For this review, take the finished solid that the model builds, in its own axes (mm). A direction names the side the tool comes from. Round coordinates to 2 decimals unless told otherwise and drop trailing zeros. Write each loop counter-clockwise with the first axis right and the second up, starting at its lowest first coordinate (ties: lowest second). Pieces come first, ordered by that corner, then holes.
from build123d import *

# Parameters (mm, degrees)
F1_DEPTH = 50.8
F2_DEPTH = 18.288
F3_DEPTH = 6.35
F0_W     = 25.4
F0_H     = 38.6286331601
F5_R     = 5.08


with BuildPart() as f1:
    # F0 (on Front) → F1 (new body, symmetric)
    with BuildSketch(Plane.XZ):
        Polygon((38.1, -12.7), (38.1, 12.7), (16.5100004677, 12.7), (-30.6439399719, 12.7), (-38.1, 12.7), (-38.1, -12.7), align=None)
    extrude(amount=F1_DEPTH, both=True)

    # F0 (on Front) → F2 (join, symmetric)
    with BuildSketch(Plane.XZ):
        with BuildLine():
            Line((16.5100004677, 12.7), (38.1, 12.7))
            Line((38.1, 12.7), (38.1, 24.0545344999))
            ThreePointArc((38.1, 24.0545344999), (39.9923105597, 28.6229763174), (44.5607523772, 30.5152868771))
            Line((44.5607523772, 30.5152868771), (51.4560379088, 30.5152868771))
            Line((51.4560379088, 30.5152868771), (51.4560379088, 52.1052864094))
            Line((51.4560379088, 52.1052864094), (44.5607523772, 52.1052864094))
            ThreePointArc((44.5607523772, 52.1052864094), (24.7258754846, 43.8894113925), (16.5100004677, 24.0545344999))
            Line((16.5100004677, 24.0545344999), (16.5100004677, 12.7))
        make_face()
        Polygon((51.4560379088, 52.1052864094), (51.4560379088, 30.5152868771), (64.020066675, 30.5152868771), (64.020066675, 52.1052864094), (58.4391281009, 52.1052864094), align=None)
    extrude(amount=F2_DEPTH, both=True)

    # F0 (on Front) → F3 (join, symmetric)
    with BuildSketch(Plane.XZ):
        with BuildLine():
            Line((-30.6439399719, 12.7), (16.5100004677, 12.7))
            Line((16.5100004677, 12.7), (16.5100004677, 24.0545344999))
            ThreePointArc((16.5100004677, 24.0545344999), (24.7258754846, 43.8894113925), (44.5607523772, 52.1052864094))
            Line((44.5607523772, 52.1052864094), (51.4560379088, 52.1052864094))
            Line((51.4560379088, 52.1052864094), (51.4560379088, 56.1626598461))
            add(Edge.make_bspline(
                [(51.4560379088, 56.1626598461), (40.4668177648, 57.3816540823), (15.1828966136, 61.2777253632), (-18.425734597, 32.7653036797), (-26.9961953148, 18.7397968243), (-30.6439399719, 12.7)],
                knots=[0.062706619, 0.062706619, 0.062706619, 0.062706619, 0.3573556866, 0.7280176576, 1, 1, 1, 1], degree=3))
        make_face()
        with BuildLine():
            add(Edge.make_bspline(
                [(58.4391281009, 55.5037148297), (56.1240075207, 55.6667510787), (53.7947415268, 55.9032359568), (51.4560379088, 56.1626598461)],
                knots=[0, 0, 0, 0, 0.062706619, 0.062706619, 0.062706619, 0.062706619], degree=3))
            Line((51.4560379088, 56.1626598461), (51.4560379088, 52.1052864094))
            Line((51.4560379088, 52.1052864094), (58.4391281009, 52.1052864094))
            Line((58.4391281009, 52.1052864094), (58.4391281009, 55.5037148297))
        make_face()
    extrude(amount=F3_DEPTH, both=True)

    # F0 (on Front) → F4 (revolve)
    with BuildSketch(Plane.XZ):
        with Locations((89.5560379088, 39.5638855255)):
            Rectangle(F0_W, F0_H)
    revolve(axis=Axis((76.8560379088, 0, 39.5638855255), (0, 0, -1)))

    # F5
    f5_edges = [f1.edges().sort_by_distance(p)[0] for p in [
        (-38.1, 0, 12.7),
        (0, -50.8, 12.7),
        (38.1, -34.544, 12.7),
        (38.1, -50.8, 0),
        (-38.1, -50.8, 0),
        (38.1, 34.544, 12.7),
        (38.1, 50.8, 0),
        (0, 50.8, 12.7),
        (-38.1, 50.8, 0),
    ]]
    fillet(f5_edges, radius=F5_R)


solid = f1.part
(1) We need section A-A, the plane z = 0. Give the boundary of the cut face in (x, y).
Geometry check:
outline: (-38.1, -45.72) arc R5.08 ccw to (-33.02, -50.8) - (33.02, -50.8) arc R5.08 ccw to (38.1, -45.72) - (38.1, 45.72) arc R5.08 ccw to (33.02, 50.8) - (-33.02, 50.8) arc R5.08 ccw to (-38.1, 45.72) - close
(2) For pin 1 Ø4 at (x, z) = (73.5, 42) entering from -Y; pin 2 Ø22.5 at (x, z) = (23, 38.5) entering from +Y; pin 3 Ø2 at (y, z) = (2.5, -2) entering from +X, all flat-tipped, find the tip position at first contact; note any pin that passes through.
Geometry check:
pin 1: stops at y = -25.36
pin 2: stops at y = 18.29
pin 3: stops at x = 38.1
(3) We need section B-B, the plane y = -9.5. Give the boundary of the cut face in (x, z), and give its area (3 significant figures).
Geometry check:
outline: (-38.1, -12.7) - (38.1, -12.7) - (38.1, 24.05) arc R6.46 cw to (44.56, 30.52) - (53.3, 30.52) - (53.3, 20.25) - (100.41, 20.25) - (100.41, 58.88) - (53.3, 58.88) - (53.3, 52.11) - (44.56, 52.11) arc R28.05 ccw to (16.51, 24.05) - (16.51, 12.7) - (-33.02, 12.7) arc R5.08 ccw to (-38.1, 7.62) - close
area: 4,770 mm2
(4) For line 1 along Z through (x, y) = (1, -37); line 2 along X through (y, z) = (1.5, -6.5); line 3 along Z through (x, y) = (92.5, -1), list the stretches that pass through material, from the lowest coordinate up.
Geometry check:
line 1: z = -12.7 to 12.7
line 2: x = -38.1 to 38.1
line 3: z = 20.25 to 58.88
(5) Mouldability with a two-part tool opening along X and no side actions: class faces 1 (the face through (24.95, 12.24, 44.11)), 2 (the face through (50, 0, 30.515)), 3 (the face through (10, -6.35, 32)), 4 (the face through (36.651, -49.272, -2.398)) as pulls with the +X half, pulls with the -X half, needs draft (parallel to the pull), parting line crosses it, or undercut.
Geometry check:
face 1: pulls with the -X half
face 2: undercut
face 3: needs draft
face 4: pulls with the +X half
(6) We need section C-C, the plane x = 80. Give the boundary of the cut face in (y, z), and give its area (3 significant figures).
Geometry check:
outline: (-25.2, 20.25) - (25.2, 20.25) - (25.2, 58.88) - (-25.2, 58.88) - close
area: 1,950 mm2
(7) For faces 5 (the face through (-36.572, 49.351, -2.682)), 6 (the face through (77, 0, 20.25)), 7 (the face through (16.51, 12, 18)), 8 (the face through (50, -14, 52.105)), 9 (the face through (-0.462, -49.272, 11.251)), list the 3-axis set-ups (+Z, -Z, +X, -X, +Y, -Y) from which the entire face can be reached by the end or side of a thin tool; tool diameter is ignored.
Geometry check:
face 5: +Z, -Z, -X, +Y
face 6: -Z, +X, +Y, -Y
face 7: +Z, -X, +Y
face 8: +Z, -X, -Y
face 9: +Z, +X, -X, -Y
